Here's how the part is built. I have some questions about the finished solid (model axes, mm). A direction names the side the tool comes from. Round coordinates to 2 decimals unless told otherwise and drop trailing zeros. Order: outer loops, then holes, each group sorted by start corner. A loop starts at its lowest first (then second) coordinate and runs counter-clockwise, first axis right, second up. Notation, with made-up numbers: (67.25, -15) -> (71.25, -15) arc R23 ccw to (71.25, 16) -> close; hole circle Ø6 at (-38.75, 73). An arc over 180 degrees is marked (long way). Use a Markdown table: item, result. Add a question column.
(1) I want a section at B-B, the plane y = 0.95. Give the number of separate pieces and of enclosed holes in the cut face, then the cut area to 3 significant figures.
(2) Thinking about a two-plate mould opening in X: for faces 1 (the face through (-0.304, 1.232, 5.478)), 2 (the face through (5, 1, -2)), 3 (the face through (-6.81, 1.02, -1.77)), which applies, pulls with the +X half, pulls with the -X half, needs draft (parallel to the pull), parting line crosses it, or undercut?
(3) I want a section at A-A, the plane x = 4.5. Please give me the cut outline in (y, z).
(4) I'm going to push flat-ended pins straight in: P1, Ø2, axis at x = -4, y = 2, coming from the +Z side; P2, Ø1.5, axis at x = -1.5, y = 1, coming from the +Z side; P3, Ø1, axis at x = 4, y = 2.5, coming from the +Z side. Where does each tip first touch, or does it pass through?
(5) On a 3-axis mill with a long thin cutter (end or side, diameter ignored), from which of +Z, -Z, +X, -X, +Y, -Y can I reach the whole of each face in a straight line? I mean faces 4 (the face through (-2, 1, 5)), 5 (the face through (-2, 1, -5)), 6 (the face through (-5.38, 1.23, -0.07)). Say none if no direction works.
(6) If I drill on probe 1 along X at (y, z) = (-0.1, 6.25); probe 2 along Y at (x, z) = (1, -3.5); probe 3 along X at (y, z) = (1.05, 6), over which ranges is the centre line in solid material (lowest first)?
from build123d import *

# Parameters (mm, degrees)
BOSS_EXTRUDE1_DEPTH                             = 2.5
BOSS_EXTRUDE1_DEPTH_BACK                        = 0.5
BOSS_EXTRUDE2_DEPTH                             = 0.5
FILLET1_R                                       = 1
CUT_EXTRUDE1_START                              = -3
SKETCH5_R                                       = 0.5
CUT_EXTRUDE1_DEPTH                              = 3
SKETCH10_W                                      = 1
SKETCH10_H                                      = 3.75
SKETCH10_W_2                                    = 3.75
SKETCH10_H_2                                    = 1
CUT_EXTRUDE2_DEPTH                              = 0.5
SKETCH17_R                                      = 1.5
BOSS_EXTRUDE3_DEPTH                             = 0.5
CSK_FOR_M2_FLAT_HEAD_MACHINE_SCREW1_D           = 2.4
CSK_FOR_M2_FLAT_HEAD_MACHINE_SCREW1_DEPTH       = 6
CSK_FOR_M2_FLAT_HEAD_MACHINE_SCREW1_CSINK_D     = 4.4
CSK_FOR_M2_FLAT_HEAD_MACHINE_SCREW1_CSINK_ANGLE = 90
CSK_FOR_M2_FLAT_HEAD_MACHINE_SCREW1_TIP         = 0.721032743
FILLET2_R                                       = 2
FILLET3_R                                       = 1


with BuildPart() as part:
    # Sketch3 → Boss-Extrude1 (new, two sides: drawn at the far end of the back side and taken through both)
    with BuildSketch(Plane(origin=(0, 0, 0), x_dir=(1, 0, 0), z_dir=(0, 1, 0)).offset(-BOSS_EXTRUDE1_DEPTH_BACK)):
        with BuildLine():
            Line((-2, -6.968679932), (-2, -2))
            Line((-2, -2), (-6.968679932, -2))
            ThreePointArc((-6.968679932, -2), (-7.179325508, -1.009844169), (-7.25, 0))
            ThreePointArc((-7.25, 0), (-7.179325508, 1.009844169), (-6.968679932, 2))
            Line((-6.968679932, 2), (-2, 2))
            Line((-2, 2), (-2, 6.968679932))
            ThreePointArc((-2, 6.968679932), (-1.009844169, 7.179325508), (0, 7.25))
            ThreePointArc((0, 7.25), (1.009844169, 7.179325508), (2, 6.968679932))
            Line((2, 6.968679932), (2, 2))
            Line((2, 2), (6.968679932, 2))
            ThreePointArc((6.968679932, 2), (7.179325508, 1.009844169), (7.25, 0))
            ThreePointArc((7.25, 0), (7.179325508, -1.009844169), (6.968679932, -2))
            Line((6.968679932, -2), (2, -2))
            Line((2, -2), (2, -6.968679932))
            ThreePointArc((2, -6.968679932), (1.009844169, -7.179325508), (0, -7.25))
            ThreePointArc((0, -7.25), (-1.009844169, -7.179325508), (-2, -6.968679932))
        make_face()
    extrude(amount=BOSS_EXTRUDE1_DEPTH + BOSS_EXTRUDE1_DEPTH_BACK)

    # Sketch4 → Boss-Extrude2 (add)
    with BuildSketch(Plane(origin=(0, 2.5, 0), x_dir=(-1, 0, 0), z_dir=(0, 1, 0))):
        with BuildLine():
            Line((-0.5, 5.875), (-0.5, 7.232738071))
            ThreePointArc((-0.5, 7.232738071), (0, 7.25), (0.5, 7.232738071))
            Line((0.5, 7.232738071), (0.5, 5.875))
            ThreePointArc((0.5, 5.875), (0, 5.375), (-0.5, 5.875))
        make_face()
        with BuildLine():
            Line((0.5, 3.125), (0.5, 0.5))
            Line((0.5, 0.5), (3.125, 0.5))
            ThreePointArc((3.125, 0.5), (3.625, 0), (3.125, -0.5))
            Line((3.125, -0.5), (0.5, -0.5))
            Line((0.5, -0.5), (0.5, -3.125))
            ThreePointArc((0.5, -3.125), (0, -3.625), (-0.5, -3.125))
            Line((-0.5, -3.125), (-0.5, -0.5))
            Line((-0.5, -0.5), (-3.125, -0.5))
            ThreePointArc((-3.125, -0.5), (-3.625, 0), (-3.125, 0.5))
            Line((-3.125, 0.5), (-0.5, 0.5))
            Line((-0.5, 0.5), (-0.5, 3.125))
            ThreePointArc((-0.5, 3.125), (0, 3.625), (0.5, 3.125))
        make_face()
        with BuildLine():
            Line((5.875, 0.5), (7.232738071, 0.5))
            ThreePointArc((7.232738071, 0.5), (7.25, 0), (7.232738071, -0.5))
            Line((7.232738071, -0.5), (5.875, -0.5))
            ThreePointArc((5.875, -0.5), (5.375, 0), (5.875, 0.5))
        make_face()
        with BuildLine():
            Line((0.5, -5.875), (0.5, -7.232738071))
            ThreePointArc((0.5, -7.232738071), (0, -7.25), (-0.5, -7.232738071))
            Line((-0.5, -7.232738071), (-0.5, -5.875))
            ThreePointArc((-0.5, -5.875), (0, -5.375), (0.5, -5.875))
        make_face()
        with BuildLine():
            Line((-5.875, -0.5), (-7.232738071, -0.5))
            ThreePointArc((-7.232738071, -0.5), (-7.25, 0), (-7.232738071, 0.5))
            Line((-7.232738071, 0.5), (-5.875, 0.5))
            ThreePointArc((-5.875, 0.5), (-5.375, 0), (-5.875, -0.5))
        make_face()
    extrude(amount=BOSS_EXTRUDE2_DEPTH)

    # Fillet1
    fillet1_edges = [part.edges().sort_by_distance(p)[0] for p in [
        (-2, 1, 6.968679932),
        (-6.968679932, 1, 2),
        (-6.968679932, 1, -2),
        (-2, 1, -6.968679932),
        (2, 1, -6.968679932),
        (6.968679932, 1, -2),
        (6.968679932, 1, 2),
        (2, 1, 6.968679932),
    ]]
    fillet(fillet1_edges, radius=FILLET1_R)

    # Sketch5 → Cut-Extrude1 (cut)
    with BuildSketch(Plane(origin=(0, 3, 0), x_dir=(-1, 0, 0), z_dir=(0, 1, 0)).offset(CUT_EXTRUDE1_START)):
        with Locations(Location((0, 5.875, 0), (0, 0, 90))):
            Circle(SKETCH5_R)
        with Locations(Location((0, 3.125, 0), (0, 0, 90))):
            Circle(SKETCH5_R)
        with Locations(Location((5.875, 0, 0), (0, 0, 90))):
            Circle(SKETCH5_R)
        with Locations(Location((3.125, 0, 0), (0, 0, 90))):
            Circle(SKETCH5_R)
        with Locations(Location((0, -5.875, 0), (0, 0, 90))):
            Circle(SKETCH5_R)
        with Locations(Location((0, -3.125, 0), (0, 0, 90))):
            Circle(SKETCH5_R)
        with Locations(Location((-5.875, 0, 0), (0, 0, 90))):
            Circle(SKETCH5_R)
        with Locations(Location((-3.125, 0, 0), (0, 0, 90))):
            Circle(SKETCH5_R)
    extrude(amount=CUT_EXTRUDE1_DEPTH, mode=Mode.SUBTRACT)

    # Sketch10 → Cut-Extrude2 (cut)
    with BuildSketch(Plane(origin=(0, 3, 0), x_dir=(1, 0, 0), z_dir=(0, 1, 0))):
        with Locations((0, -4.5)):
            Rectangle(SKETCH10_W, SKETCH10_H)
        with Locations((-4.5, 0)):
            Rectangle(SKETCH10_W_2, SKETCH10_H_2)
        with Locations((0, 4.5)):
            Rectangle(SKETCH10_W, SKETCH10_H)
        with Locations((4.5, 0)):
            Rectangle(SKETCH10_W_2, SKETCH10_H_2)
    extrude(amount=-CUT_EXTRUDE2_DEPTH, mode=Mode.SUBTRACT)

    # Sketch17 → Boss-Extrude3 (add)
    with BuildSketch(Plane(origin=(0, 2.5, 0), x_dir=(1, 0, 0), z_dir=(0, 1, 0))):
        Circle(SKETCH17_R)
    extrude(amount=BOSS_EXTRUDE3_DEPTH)

    # CSK for M2 Flat Head Machine Screw1
    with Locations(Plane(origin=(0, -0.5, 0), x_dir=(-1, 0, 0), z_dir=(0, -1, 0))):
        with Locations((0, 0)):
            CounterSinkHole(CSK_FOR_M2_FLAT_HEAD_MACHINE_SCREW1_D / 2, CSK_FOR_M2_FLAT_HEAD_MACHINE_SCREW1_CSINK_D / 2, depth=CSK_FOR_M2_FLAT_HEAD_MACHINE_SCREW1_DEPTH, counter_sink_angle=CSK_FOR_M2_FLAT_HEAD_MACHINE_SCREW1_CSINK_ANGLE)
            with Locations((0, 0, -(CSK_FOR_M2_FLAT_HEAD_MACHINE_SCREW1_DEPTH + CSK_FOR_M2_FLAT_HEAD_MACHINE_SCREW1_TIP / 2))):  # 118° drill point
                Cone(0, CSK_FOR_M2_FLAT_HEAD_MACHINE_SCREW1_D / 2, CSK_FOR_M2_FLAT_HEAD_MACHINE_SCREW1_TIP, mode=Mode.SUBTRACT)

    # Fillet2
    fillet2_edges = [part.edges().sort_by_distance(p)[0] for p in [
        (-2, 1, 2),
        (-2, 1, -2),
        (2, 1, -2),
        (2, 1, 2),
    ]]
    fillet(fillet2_edges, radius=FILLET2_R)

    # Fillet3
    fillet3_edges = [part.edges().sort_by_distance(p)[0] for p in [
        (0.5, 2.75, 1.414213562),
        (1.414213562, 2.75, 0.5),
        (1.414213562, 2.75, -0.5),
        (0.5, 2.75, -1.414213562),
        (-0.5, 2.75, -1.414213562),
        (-1.414213562, 2.75, -0.5),
        (-1.414213562, 2.75, 0.5),
        (-0.5, 2.75, 1.414213562),
    ]]
    fillet(fillet3_edges, radius=FILLET3_R)


solid = part.part
Taken from the geometry:
| question | item | result |
|---|---|---|
| 1 | separate pieces | 1 |
| 1 | enclosed holes | 9 |
| 1 | area | 90.1 mm2 |
| 2 | face 1 | undercut |
| 2 | face 2 | needs draft |
| 2 | face 3 | pulls with the -X half |
| 3 | outline | (-0.5, -2) -> (2.5, -2) -> (2.5, 2) -> (-0.5, 2) -> close |
| 4 | P1 | stops at z = 2.27 |
| 4 | P2 | stops at z = 7.21 |
| 4 | P3 | stops at z = 2.06 |
| 5 | face 4 | +Z, -X, +Y, -Y |
| 5 | face 5 | -Z, -X, +Y, -Y |
| 5 | face 6 | +Y |
| 6 | probe 1 | x = -2 to 2 |
| 6 | probe 2 | y = -0.5 to 2.5 |
| 6 | probe 3 | x = -2 to -0.48, 0.48 to 2 |
